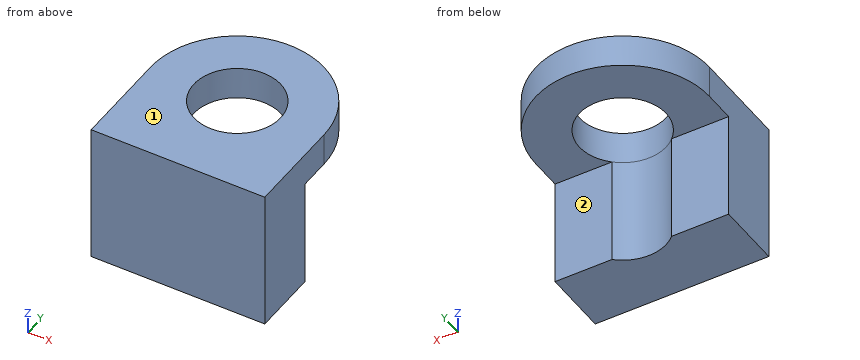
```python
from build123d import *

# Parameters (mm, degrees)
SKETCH1_R           = 40
SKETCH1_R_2         = 20
BOSS_EXTRUDE1_DEPTH = 15
BOSS_EXTRUDE2_START = 50
BOSS_EXTRUDE2_DEPTH = 50


with BuildPart() as part:
    # Sketch1 → Boss-Extrude1 (new body)
    # profile 1 of 2: a face of its own
    with BuildSketch(Plane.XY):
        Circle(SKETCH1_R)
        Circle(SKETCH1_R_2, mode=Mode.SUBTRACT)
    # profile 2 of 2: a face of its own
    with BuildSketch(Plane.XY):
        with BuildLine():
            ThreePointArc((40, 0), (0, -40), (-40, 0))
            Line((-40, 0), (-40, -45))
            Line((-40, -45), (40, -45))
            Line((40, -45), (40, 0))
        make_face()
    extrude(amount=BOSS_EXTRUDE1_DEPTH)

    # Sketch3 → Boss-Extrude2 (add)
    with BuildSketch(Plane(origin=(0, 0, 0), x_dir=(-1, 0, 0), z_dir=(0, 0, -1)).offset(BOSS_EXTRUDE2_START)):
        with BuildLine():
            Line((13.774977314, -14.5), (40, -14.5))
            Line((40, -14.5), (40, -45))
            Line((40, -45), (-40, -45))
            Line((-40, -45), (-40, -14.5))
            Line((-40, -14.5), (-13.774977314, -14.5))
            ThreePointArc((-13.774977314, -14.5), (0, -20), (13.774977314, -14.5))
        make_face()
    extrude(amount=-BOSS_EXTRUDE2_DEPTH)


solid = part.part
```
Check sheet for the modelled part. Datum: model origin and axes. Units: mm. Face numbers are marked on the shaded views. A direction names the side the tool comes from. Round coordinates to 2 decimals unless told otherwise and drop trailing zeros. Order: outer loops, then holes, each group sorted by start corner. A loop starts at its lowest first (then second) coordinate and runs counter-clockwise, first axis right, second up. Notation, with made-up numbers: (60.5, -22.75) -> (77.5, -22.75) arc R24 ccw to (77.5, 15.25) -> close; hole circle Ø8 at (49.25, 76). An arc over 180 degrees is marked (long way). Use CSV: the item, a comma, the result in double quotes.
(1) Cross-section at C-C (z = -33). Record the boundary of the cut face in (x, y).
Worked out:
outline,"(-40, -45) -> (40, -45) -> (40, -14.5) -> (13.77, -14.5) arc R20 cw to (-13.77, -14.5) -> (-40, -14.5) -> close"
(2) Material ranges on line 1 along X through (y, z) = (0, 9.5); line 2 along Y through (x, z) = (0, 4.25); line 3 along Z through (x, y) = (32.5, 22.5), recorded low to high. Write a range as from..to.
Worked out:
line 1,"-40..-20, 20..40"
line 2,"-45..-20, 20..40"
line 3,"0..15"
(3) Depth check by flat-ended pin: pin 1 (1 mm diameter, centred on x = -19.5, z = 1, fed in from +Y); pin 2 (10 mm diameter, centred on x = -27, z = -23.5, fed in from +Y); pin 3 (16.5 mm diameter, centred on x = 14, y = -0.5, fed in from -Z). Enter the tip coordinate at first touch or a pass-through.
Worked out:
pin 1,"y = 35.2"
pin 2,"y = -14.5"
pin 3,"z = 0"
(4) Cross-section at D-D (y = 32.5). Record the boundary of the cut face in (x, z).
Worked out:
outline,"(-23.32, 0) -> (23.32, 0) -> (23.32, 15) -> (-23.32, 15) -> close"
(5) Cross-section at A-A (x = 0). Record the boundary of the cut face in (y, z).
Worked out:
outline,"(-45, -50) -> (-20, -50) -> (-20, 15) -> (-45, 15) -> close; (20, 0) -> (40, 0) -> (40, 15) -> (20, 15) -> close"
(6) Cross-section at B-B (y = 7.5). Record the boundary of the cut face in (x, z), and give its area (3 significant figures).
Worked out:
outline,"(-39.29, 0) -> (-18.54, 0) -> (-18.54, 15) -> (-39.29, 15) -> close; (18.54, 0) -> (39.29, 0) -> (39.29, 15) -> (18.54, 15) -> close"
area,"623 mm²"
(7) Tool access check on the marked faces 1 and 2. Record the directions out of +Z, -Z, +X, -X, +Y, -Y that give a thin tool (end or side, any length) a straight path to the whole face; none if there is none.
Worked out:
face 1,"+Z, +X, -X, +Y, -Y"
face 2,"-Z, +X, -X, +Y"
